```python
from build123d import *

# Parameters (mm, degrees)
F0_R     = 5.55625
F1_DEPTH = 6.35


with BuildPart() as f1:
    # F0 (on Front) → F1 (new body)
    with BuildSketch(Plane.XZ):
        with BuildLine():
            ThreePointArc((9.890924, 38.017616), (4.981184, 38.918746), (-0.001432, 39.220595))
            ThreePointArc((-0.001432, 39.220595), (-4.984048, 38.918746), (-9.893787, 38.017616))
            Line((-9.893787, 38.017616), (-100.420647, 15.669758))
            ThreePointArc((-100.420647, 15.669758), (-114.301432, -2.054405), (-100.420647, -19.778569))
            Line((-100.420647, -19.778569), (-9.893787, -42.126427))
            ThreePointArc((-9.893787, -42.126427), (-0.001769, -43.329405), (9.89027, -42.126589))
            Line((9.89027, -42.126589), (100.423844, -19.77864))
            ThreePointArc((100.423844, -19.77864), (114.304918, -2.054405), (100.423844, 15.669829))
            Line((100.423844, 15.669829), (9.890924, 38.017616))
        make_face()
        with BuildLine():
            ThreePointArc((-65.088932, -2.054405), (-59.532682, 3.501845), (-53.976432, -2.054405))
            ThreePointArc((-53.976432, -2.054405), (-59.532682, -7.610655), (-65.088932, -2.054405))
        make_face(mode=Mode.SUBTRACT)
        with BuildLine():
            ThreePointArc((-0.001432, 26.520595), (20.204145, 18.151171), (28.573568, -2.054405))
            ThreePointArc((28.573568, -2.054405), (-20.207008, -22.259982), (-0.001432, 26.520595))
        make_face(mode=Mode.SUBTRACT)
        with Locations((59.536168, -2.054405)):
            Circle(F0_R, mode=Mode.SUBTRACT)
    extrude(amount=F1_DEPTH)


solid = f1.part
```
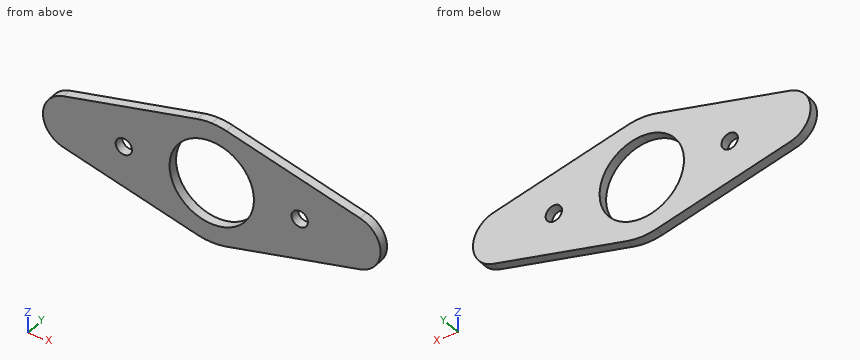
Part model, mm, in its own coordinate system. Round coordinates to 2 decimals unless told otherwise and drop trailing zeros. Write each loop counter-clockwise with the first axis right and the second up, starting at its lowest first coordinate (ties: lowest second). Pieces come first, ordered by that corner, then holes. Notation, with made-up numbers: (9, 14) -> (55, 14) arc R22 ccw to (55, 41) -> close; hole circle Ø4 at (-22.75, -18). An arc over 180 degrees is marked (long way). Return JSON: item names as keys, results as strings. Group by question number.
Q1. Saw through at B-B on x = -17.5. Write the cut outline in (y, z), plus the area to 3 significant figures.
Q2. Pin check, flat tip, straight feed: pin 1 (2 mm diameter, centred on y = -0.5, z = 0, fed in from +X). Stop position of the tip, or through.
Q3. Saw through at A-A on z = 23. Write the cut outline in (x, y), plus the area to 3 significant figures.
Q4. Saw through at C-C on y = -4. State how many separate pieces and enclosed holes the cut face has, plus the area to 3 significant figures.
Q5. Saw through at D-D on z = -4.5. Write the cut outline in (x, y), plus the area to 3 significant figures.
Q6. Probe L1, parallel to X at y = -3.5, z = 3; L2, parallel to Z at x = 14, y = -1.25; L3, parallel to Z at x = -9.5, y = -0.25. List the from-to ranges inside material, lowest first. Write a range as [from, to].
Answer:
{
 "1": {"outline": "(-6.35, -40.25) -> (0, -40.25) -> (0, -24.64) -> (-6.35, -24.64) -> close; (-6.35, 20.54) -> (0, 20.54) -> (0, 36.14) -> (-6.35, 36.14) -> close", "area": "198 mm2"},
 "2": {"pin 1": "x = 114.27"},
 "3": {"outline": "(-70.73, -6.35) -> (-13.74, -6.35) -> (-13.74, 0) -> (-70.73, 0) -> close; (13.74, -6.35) -> (70.73, -6.35) -> (70.73, 0) -> (13.74, 0) -> close", "area": "724 mm2"},
 "4": {"separate pieces": "1", "enclosed holes": "3", "area": "10,100 mm2"},
 "5": {"outline": "(-114.14, -6.35) -> (-64.52, -6.35) -> (-64.52, 0) -> (-114.14, 0) -> close; (-54.54, -6.35) -> (-28.47, -6.35) -> (-28.47, 0) -> (-54.54, 0) -> close; (28.47, -6.35) -> (54.55, -6.35) -> (54.55, 0) -> (28.47, 0) -> close; (64.53, -6.35) -> (114.14, -6.35) -> (114.14, 0) -> (64.53, 0) -> close", "area": "961 mm2"},
 "6": {"L1": "[-113.59, -61.84], [-57.23, -28.13], [28.12, 57.23], [61.84, 113.59]", "L2": "[-41.11, -26.96], [22.86, 37]", "L3": "[-42.22, -29], [24.9, 38.11]"}
}
